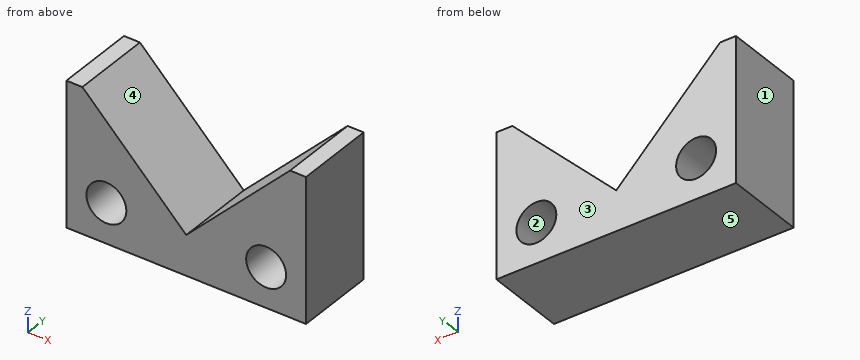
Autodesk Inventor part; units mm, degrees
ref_plane "YZ Plane" through (0, 0, 0) normal (1, 0, 0) x (0, 1, 0)
ref_plane "XZ Plane" through (0, 0, 0) normal (0, 1, 0) x (-1, 0, 0)
ref_plane "XY Plane" through (0, 0, 0) normal (0, 0, 1) x (1, 0, 0)
sketch "Boceto1" plane through (0, 0, 0) normal (0, 1, 0) x (-1, 0, 0)
  line L0 (-15, -10) -> (15, -10)
  line L1 (13, 8) -> (0, -5)
  line L2 (-13, 8) -> (0, -5)
  line L3 (-15, 8) -> (-13, 8)
  line L4 (15, 8) -> (13, 8)
  line L5 (15, -10) -> (15, 8)
  line L6 (-15, -10) -> (-15, 8)
  line L7 (15, -10) -> (10, -10)
  line L8 (-15, -10) -> (-10, -10)
  circle A0 centre (-10, -5) radius 2.5
  circle A1 centre (10, -5) radius 2.5
  point P0 (0, 0)
  dimension "d5" = 5
  dimension "d8" = 5
  dimension "d9" = 5
extrude "Extrusión1" add sketch "Boceto1" along normal blind 10
properties part number "_3DPrint"
Design review of the part built by this model. Coordinates are the model's own, in mm. Face numbers are marked on the shaded views. A direction names the side the tool comes from. Round coordinates to 2 decimals unless told otherwise and drop trailing zeros. Loops run counter-clockwise (first coordinate to the right, second up) from the corner with the lowest first, then second, coordinate; pieces in that order, holes last. Notation, with made-up numbers: (80, 23.25) - (107, 23.25) arc R12 cw to (107, 45.25) - close; hole circle Ø4 at (54, -33). An arc over 180 degrees is marked (long way). One line per question, with ' | ' between items.
1. We need section D-D, the plane z = -3. State the section outline as (x, y) points, and give its area (3 significant figures).
Results are:
outline: (-15, 0) - (-11.5, 0) - (-11.5, 10) - (-15, 10) - close; (-8.5, 0) - (-2, 0) - (-2, 10) - (-8.5, 10) - close; (2, 0) - (8.5, 0) - (8.5, 10) - (2, 10) - close; (11.5, 0) - (15, 0) - (15, 10) - (11.5, 10) - close | area: 200 mm²
2. Clearance check with flat-ended pins moving along their axes: P1, Ø6.5, axis at x = -10, z = -5, coming from the -Y side; P2, Ø1.5, axis at x = -11.5, y = 8.5, coming from the +Z side. State where each tip first meets the part, or that it passes through.
Results are:
P1: stops at y = 0 | P2: stops at z = 7.25
3. For the marked faces 4 and 5, list the 3-axis set-ups (+Z, -Z, +X, -X, +Y, -Y) from which the entire face can be reached by the end or side of a thin tool; tool diameter is ignored.
Results are:
face 4: +Z, +Y, -Y | face 5: -Z, +X, -X, +Y, -Y
4. We need section B-B, the plane x = -10. State the section outline as (y, z) points.
Results are:
outline: (0, -10) - (10, -10) - (10, -7.5) - (0, -7.5) - close; (0, -2.5) - (10, -2.5) - (10, 5) - (0, 5) - close
5. For L1, parallel to X at y = 3, z = -5.75; L2, parallel to Z at x = 5, y = 4.25; L3, parallel to X at y = 0.75, z = 4.5, list the stretches that pass through material, from the lowest coordinate up. Write a range as [from, to].
Results are:
L1: x = [-15, -12.38], [-7.62, 7.62], [12.38, 15] | L2: z = [-10, 0] | L3: x = [-15, -9.5], [9.5, 15]
6. We need section A-A, the plane z = 1.5. State the section outline as (x, y) points.
Results are:
outline: (-15, 0) - (-6.5, 0) - (-6.5, 10) - (-15, 10) - close; (6.5, 0) - (15, 0) - (15, 10) - (6.5, 10) - close
7. We need section C-C, the plane y = 5.5. State the section outline as (x, z) points.
Results are:
outline: (-15, -10) - (15, -10) - (15, 8) - (13, 8) - (0, -5) - (-13, 8) - (-15, 8) - close; hole circle Ø5 at (-10, -5); hole circle Ø5 at (10, -5)
8. Draft analysis for pull direction X (two halves, no side actions). For the marked faces 1, 2 and 3, state which applies: released by +X, released by -X, zero draft, split by the parting line, or undercut.
Results are:
face 1: released by -X | face 2: undercut | face 3: zero draft
